Autodesk Inventor part; units mm, degrees
ref_plane "Work Plane1" through (0, 0, 0) normal (0, 0, 1) x (1, 0, 0)
ref_plane "YZ Plane" through (0, 0, 0) normal (1, 0, 0) x (0, 1, 0)
ref_plane "XZ Plane" through (0, 0, 0) normal (0, 1, 0) x (-1, 0, 0)
ref_plane "Work Plane1" through (0, 0, 0) normal (0, 0, 1) x (1, 0, 0)
sketch "Sketch1" plane through (0, 0, 0) normal (0, 0, 1) x (1, 0, 0)
  line L0 (-200, 125) -> (70, 125)
  line L1 (-200, -125) -> (-200, 125)
  line L2 (180, -125) -> (-200, -125)
  line L3 (180, 15) -> (180, -125)
  arc A0 (180, 15) -> (70, 125) centre (70, 15) ccw
  point P0 (0, 0)
extrude "Plate1" add sketch "Sketch1" against normal blind 1.5
equation "\"d0\" = Thickness"
equation "\"BendRadius\" = Thickness"
equation "\"BendReliefWidth\" = Thickness"
equation "\"BendReliefDepth\" = 0.5 * Thickness"
equation "\"CornerReliefSize\" = 4 * Thickness"
equation "\"MinimumRemnant\" = 2 * Thickness"
equation "\"TransitionRadius\" = BendRadius"
equation "\"JacobiRadiusSize\" = BendRadius"
equation "\"GapSize\" = Thickness"
properties part number "CARCASA_ALUM_6"
Could you check a few things on this model? Use its own coordinates, in mm. Give positions to 0.01 mm unless a question says otherwise; leave off trailing zeros. Order: outer loops, then holes, each group sorted by start corner. A loop starts at its lowest first (then second) coordinate and runs counter-clockwise, first axis right, second up.
Q1. If I drill on line 1 along X through (y, z) = (77, -0.85); line 2 along X through (y, z) = (104.5, -1.05); line 3 along Y through (x, z) = (147, -0.8), over which ranges is the centre line in solid material (lowest first)?
Q2. Suppose I cut it at A-A, the plane z = -0.8. Write out the boundary of the cut face in (x, y).
Q3. Suppose I cut it at C-C, the plane x = 112.5. Write out the boundary of the cut face in (y, z).
Q4. Suppose I cut it at B-B, the plane y = 64. Write out the boundary of the cut face in (x, z).
Solution:
1. line 1: x = -200 to 160.86
1. line 2: x = -200 to 133.95
1. line 3: y = -125 to 93.56
2. outline: (-200, -125) - (180, -125) - (180, 15) arc R110 ccw to (70, 125) - (-200, 125) - close
3. outline: (-125, -1.5) - (116.46, -1.5) - (116.46, 0) - (-125, 0) - close
4. outline: (-200, -1.5) - (168.48, -1.5) - (168.48, 0) - (-200, 0) - close
